Verification items for the finished model (mm, model axes). A direction names the side the tool comes from. Give positions to 0.01 mm unless a question says otherwise; leave off trailing zeros. Order: outer loops, then holes, each group sorted by start corner. A loop starts at its lowest first (then second) coordinate and runs counter-clockwise, first axis right, second up. Notation, with made-up numbers: (69.5, 13) - (120.5, 13) arc R21 ccw to (120.5, 40) - close; hole circle Ø5 at (62, 46). An arc over 180 degrees is marked (long way). Answer as a JSON object with one key per item and string values.
```python
from build123d import *

# Parameters (mm, degrees)
F0_R     = 12.7
F0_R_2   = 1.968379445
F0_R_3   = 6.35
F0_R_4   = 4.0005
F1_DEPTH = 25.4
F2_DEPTH = 7.62


with BuildPart() as f1:
    # F0 (on Top) → F1 (new body)
    with BuildSketch(Plane.XY):
        Circle(F0_R)
        with Locations((0, -9.5697641373)):
            Circle(F0_R_2, mode=Mode.SUBTRACT)
        with Locations((-9.5697641373, 0)):
            Circle(F0_R_2, mode=Mode.SUBTRACT)
        Circle(F0_R_3, mode=Mode.SUBTRACT)
        with Locations((9.5697641373, 0)):
            Circle(F0_R_2, mode=Mode.SUBTRACT)
        with Locations((0, 9.5697641373)):
            Circle(F0_R_2, mode=Mode.SUBTRACT)
        Circle(F0_R_3)
        Circle(F0_R_4, mode=Mode.SUBTRACT)
    extrude(amount=F1_DEPTH)

    # F0 (on Top) → F2 (join)
    with BuildSketch(Plane.XY):
        Circle(F0_R_3)
        Circle(F0_R_4, mode=Mode.SUBTRACT)
    extrude(amount=-F2_DEPTH)


solid = f1.part
```
(1) Release check for a two-part mould opening along Y. For faces 3 (the cylindrical face through (-0.43, -11.49, 12.52)), 4 (the flat face through (-6, -3, 0)), 5 (the cylindrical face through (-2.75, -12.4, 12.52)) record: pulls with the +Y half, pulls with the -Y half, needs draft (parallel to the pull), parting line crosses it, or undercut.
Computed values:
{"face 3": "undercut", "face 4": "needs draft", "face 5": "parting line crosses it"}
(2) Section check A-A (x = 0). Record the cut outline in (y, z).
Computed values:
{"outline": "(-12.7, 0) - (-11.54, 0) - (-11.54, 25.4) - (-12.7, 25.4) - close; (-7.6, 0) - (-6.35, 0) - (-6.35, -7.62) - (-4, -7.62) - (-4, 25.4) - (-7.6, 25.4) - close; (4, -7.62) - (6.35, -7.62) - (6.35, 0) - (7.6, 0) - (7.6, 25.4) - (4, 25.4) - close; (11.54, 0) - (12.7, 0) - (12.7, 25.4) - (11.54, 25.4) - close"}
(3) Access from +Z, -Z, +X, -X, +Y, -Y to the whole of each face (thin tool, end or side, straight path). Record for faces 1 (the cylindrical face through (-1.38, -6.2, -3.76)), 2 (the flat face through (-3, 3, 25.4)).
Computed values:
{"face 1": "-Z", "face 2": "+Z, +X, -X, +Y, -Y"}
(4) Gauge pin test, flat ends, axial feed: pin 1 Ø5 at (y, z) = (7.5, 16) entering from -X; pin 2 Ø10 at (x, z) = (8, 3) entering from -Y; pin 3 Ø6.5 at (x, y) = (0, 0) entering from -Z; pin 4 Ø10 at (y, z) = (-1, 21) entering from +X. Record the tip position at first contact, or that the pin passes through.
Computed values:
{"pin 1": "stops at x = -11.67", "pin 2": "stops at y = -12.34", "pin 3": "passes through", "pin 4": "stops at x = 12.7"}
(5) Section check C-C (x = 8.75). Record the cut outline in (y, z), then the cut area to 3 significant figures.
Computed values:
{"outline": "(-9.2, 0) - (-1.79, 0) - (-1.79, 25.4) - (-9.2, 25.4) - close; (1.79, 0) - (9.2, 0) - (9.2, 25.4) - (1.79, 25.4) - close", "area": "377 mm²"}
(6) Material ranges on line 1 along Y through (x, z) = (0, 14.5); line 2 along X through (y, z) = (1, 15.5), recorded low to high. Write a range as [from, to].
Computed values:
{"line 1": "y = [-12.7, -11.54], [-7.6, -4], [4, 7.6], [11.54, 12.7]", "line 2": "x = [-12.66, -11.27], [-7.87, -3.87], [3.87, 7.87], [11.27, 12.66]"}
(7) Section check D-D (z = 5). Record the cut outline in (x, y).
Computed values:
{"outline": "circle Ø25.4 at (0, 0); hole circle Ø3.94 at (-9.57, 0); hole circle Ø8 at (0, 0); hole circle Ø3.94 at (0, -9.57); hole circle Ø3.94 at (0, 9.57); hole circle Ø3.94 at (9.57, 0)"}
